Geometry: final body of the model. Coordinates: model frame, mm. Face numbers are marked on the shaded views. A direction names the side the tool comes from. Round coordinates to 2 decimals unless told otherwise and drop trailing zeros. Write each loop counter-clockwise with the first axis right and the second up, starting at its lowest first coordinate (ties: lowest second). Pieces come first, ordered by that corner, then holes.
from build123d import *

# Parameters (mm, degrees)
EXTRUDE_1_DEPTH          = 16
CUT_EXTRUDE_1_DEPTH      = 37.249137921
CUT_EXTRUDE_1_DEPTH_BACK = 16
CUT_EXTRUDE_2_DEPTH      = 38.549966711
CUT_EXTRUDE_2_DEPTH_BACK = 16
SKETCH_4_R               = 2.5
CUT_EXTRUDE_3_DEPTH      = 16
SKETCH_5_R               = 2.5
CUT_EXTRUDE_4_DEPTH      = 16
FILLET_1_R               = 1
FILLET_2_R               = 1
CHAMFER_1_SIZE           = 1
CHAMFER_2_SIZE           = 1


with BuildPart() as part:
    # 草图1 → 凸台-拉伸1 (new body)
    with BuildSketch(Plane.XY):
        Polygon((0, 0), (0, 23), (-2, 23), (-2, -2), (23, -2), (23, 0), align=None)
    extrude(amount=EXTRUDE_1_DEPTH)

    # 草图2 → 切除-拉伸1 (cut, two sides: drawn at the far end of the back side and taken through both)
    with BuildSketch(Plane(origin=(0, 0, 0), x_dir=(0, 0, -1), z_dir=(1, 0, 0)).offset(-CUT_EXTRUDE_1_DEPTH_BACK)):
        with BuildLine():
            ThreePointArc((-16, 15), (-13.656854249, 20.656854249), (-8, 23))
            Line((-8, 23), (-16, 23))
            Line((-16, 23), (-16, 15))
        make_face()
        with BuildLine():
            ThreePointArc((-8, 23), (-2.343145751, 20.656854249), (0, 15))
            Line((0, 15), (0, 23))
            Line((0, 23), (-8, 23))
        make_face()
    extrude(amount=CUT_EXTRUDE_1_DEPTH + CUT_EXTRUDE_1_DEPTH_BACK, mode=Mode.SUBTRACT)

    # 草图3 → 切除-拉伸2 (cut, two sides: drawn at the far end of the back side and taken through both)
    with BuildSketch(Plane.XZ.offset(2).offset(-CUT_EXTRUDE_2_DEPTH_BACK)):
        with BuildLine():
            ThreePointArc((23, 8), (20.656854249, 2.343145751), (15, 0))
            Line((15, 0), (23, 0))
            Line((23, 0), (23, 8))
        make_face()
        with BuildLine():
            ThreePointArc((15, 16), (20.656854249, 13.656854249), (23, 8))
            Line((23, 8), (23, 16))
            Line((23, 16), (15, 16))
        make_face()
    extrude(amount=CUT_EXTRUDE_2_DEPTH + CUT_EXTRUDE_2_DEPTH_BACK, mode=Mode.SUBTRACT)

    # 草图4 → 切除-拉伸3 (cut)
    with BuildSketch(Plane(origin=(0, 0, 0), x_dir=(1, 0, 0), z_dir=(0, 1, 0))):
        with Locations(Location((15, -8, 0), (0, 0, 180))):
            Circle(SKETCH_4_R)
    extrude(amount=-CUT_EXTRUDE_3_DEPTH, mode=Mode.SUBTRACT)

    # 草图5 → 切除-拉伸4 (cut)
    with BuildSketch(Plane(origin=(0, 0, 0), x_dir=(0, 0, -1), z_dir=(1, 0, 0))):
        with Locations((-8, 15)):
            Circle(SKETCH_5_R)
    extrude(amount=-CUT_EXTRUDE_4_DEPTH, mode=Mode.SUBTRACT)

    # 圆角1
    fillet_1_edges = [part.edges().sort_by_distance(p)[0] for p in [
        (0, 0, 8),
    ]]
    fillet(fillet_1_edges, radius=FILLET_1_R)

    # 圆角2
    fillet_2_edges = [part.edges().sort_by_distance(p)[0] for p in [
        (-2, -2, 8),
    ]]
    fillet(fillet_2_edges, radius=FILLET_2_R)

    # 倒角1
    chamfer_1_edges = [part.edges().sort_by_distance(p)[0] for p in [
        (0, 15, 10.5),
    ]]
    chamfer(chamfer_1_edges, length=CHAMFER_1_SIZE)

    # 倒角2
    chamfer_2_edges = [part.edges().sort_by_distance(p)[0] for p in [
        (17.5, 0, 8),
    ]]
    chamfer(chamfer_2_edges, length=CHAMFER_2_SIZE)


solid = part.part
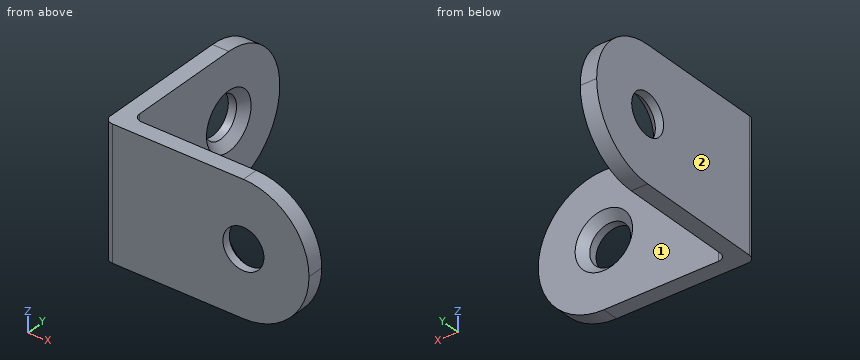
1) Section A-A on z = 14.5. Output: boundary loops of the cut face in (x, y), plus the area to 3 significant figures.
2) First-contact query: P1, Ø8, axis at y = 4.5, z = 4.5, coming from the +X side; P2, Ø5, axis at x = 11, z = 8, coming from the +Y side; P3, Ø2, axis at y = 7, z = 9, coming from the +X side; P4, Ø1.5, axis at x = 5, y = 1.5, coming from the +Z side. Flat tips, straight axial feed; report the tip coordinate or a pass-through.
3) Section D-D on z = 12.5. Output: boundary loops of the cut face in (x, y).
4) Line query: probe 1 along Z at (x, y) = (15, -1.15); probe 2 along X at (y, z) = (8.5, 9.5). Output: solid intervals per line, ascending.
5) Reachability of the marked faces 1 and 2 from +Z, -Z, +X, -X, +Y, -Y: full face, straight path, thin tool, end or side. Return the list, or none.
6) Section B-B on x = 3. Output: boundary loops of the cut face in (y, z).
Filled in:
1. outline: (-2, -1) arc R1 ccw to (-1, -2) - (19.66, -2) - (19.66, 0) - (1, 0) arc R1 cw to (0, 1) - (0, 19.66) - (-2, 19.66) - close
1. area: 82.7 mm2
2. P1: stops at x = 0.13
2. P2: stops at y = 0
2. P3: stops at x = 0
2. P4: passes through
3. outline: (-2, -1) arc R1 ccw to (-1, -2) - (21.61, -2) - (21.61, 0) - (1, 0) arc R1 cw to (0, 1) - (0, 21.61) - (-2, 21.61) - close
4. probe 1: z = 0 to 5.5, 10.5 to 16
4. probe 2: x = -2 to 0
5. face 1: +Z, -Z, +X, +Y
5. face 2: +Z, -Z, -X, +Y, -Y
6. outline: (-2, 0) - (0, 0) - (0, 16) - (-2, 16) - close
